```python
from build123d import *

# Parameters (mm, degrees)
F0_W      = 101.6
F0_H      = 76.2
F1_DEPTH  = 25.4
F2_R      = 6.35
F3_DEPTH  = 25.4
F4_W      = 25.4
F4_H      = 38.1
F6_W      = 30.48
F6_H      = 6.35
F8_R      = 5.08
F9_SIZE   = 5.08
F10_R     = 2.54
F11_SIZE  = 2.54
F12_SIZE  = 2.54
F13_R     = 10.3882483968
F14_DEPTH = 76.2


with BuildPart() as f1:
    # F0 (on Top) → F1 (new body)
    with BuildSketch(Plane.XY):
        Rectangle(F0_W, F0_H)
    extrude(amount=F1_DEPTH)

    # F2 (on face) → F3 (cut)
    with BuildSketch(Plane.XY.offset(25.4)):
        with Locations((-38.1, 25.4)):
            Circle(F2_R)
        with Locations((38.1, 25.4)):
            Circle(F2_R)
        with Locations((38.1, -25.4)):
            Circle(F2_R)
        with Locations((-38.1, -25.4)):
            Circle(F2_R)
    extrude(amount=-F3_DEPTH, mode=Mode.SUBTRACT)

    # F4 (on Front) → F5 (revolve)
    with BuildSketch(Plane.XZ):
        with Locations((-12.7, 44.45)):
            Rectangle(F4_W, F4_H)
    revolve(axis=Axis((0, 0, 44.45), (0, 0, 1)))

    # F6 (on Right) → F7 (revolve, cut)
    with BuildSketch(Plane.YZ):
        with Locations((-34.29, 41.275)):
            Rectangle(F6_W, F6_H)
    revolve(axis=Axis((0, 0, 63.5), (0, 0, -1)), mode=Mode.SUBTRACT)

    # F8
    f8_edges = [f1.edges().sort_by_distance(p)[0] for p in [
        (25.4, 0, 38.1),
    ]]
    fillet(f8_edges, radius=F8_R)

    # F9
    f9_edges = [f1.edges().sort_by_distance(p)[0] for p in [
        (0, -38.1, 25.4),
        (50.8, 0, 25.4),
        (0, 38.1, 25.4),
        (-50.8, 0, 25.4),
    ]]
    chamfer(f9_edges, length=F9_SIZE)

    # F10
    f10_edges = [f1.edges().sort_by_distance(p)[0] for p in [
        (25.4, 0, 25.4),
        (25.4, 0, 33.02),
        (25.4, 0, 44.45),
        (25.4, 0, 63.5),
    ]]
    fillet(f10_edges, radius=F10_R)

    # F11
    f11_edges = [f1.edges().sort_by_distance(p)[0] for p in [
        (0, -38.1, 0),
        (50.8, 0, 0),
        (0, 38.1, 0),
        (-50.8, 0, 0),
    ]]
    chamfer(f11_edges, length=F11_SIZE)

    # F12
    f12_edges = [f1.edges().sort_by_distance(p)[0] for p in [
        (-50.8, 38.1, 11.43),
        (-50.8, -38.1, 11.43),
        (50.8, 38.1, 11.43),
        (50.8, -38.1, 11.43),
    ]]
    chamfer(f12_edges, length=F12_SIZE)

    # F13 (on face) → F14 (cut)
    with BuildSketch(Plane.XY.offset(63.5)):
        Circle(F13_R)
    extrude(amount=-F14_DEPTH, mode=Mode.SUBTRACT)


solid = f1.part
```
Read the model definition and answer for the solid it produces. Units are mm, in the model's axes. A direction names the side the tool comes from. Coordinates: 2 decimals unless noted, no trailing zeros. Write each loop counter-clockwise with the first axis right and the second up, starting at its lowest first coordinate (ties: lowest second). Pieces come first, ordered by that corner, then holes. Notation, with made-up numbers: (-10.5, -14) -> (9.5, -14) arc R7 ccw to (9.5, -2) -> close; hole circle Ø2 at (74.5, -21). An arc over 180 degrees is marked (long way). Answer as a JSON object with one key per item and string values.
Q1. Consider line 1 (X direction, y = 25, z = 19); line 2 (Y direction, x = 38.1, z = 15.5); line 3 (Y direction, x = 0, z = 17.5). Determine where each line is inside the solid, lowest interval first. Write a range as [from, to].
The answers:
{"line 1": "x = [-50.8, -44.44], [-31.76, 31.76], [44.44, 50.8]", "line 2": "y = [-38.1, -31.75], [-19.05, 19.05], [31.75, 38.1]", "line 3": "y = [-38.1, -10.39], [10.39, 38.1]"}
Q2. Flat-ended cylindrical pins translate along their axes: pin 1 Ø16.5 at (x, y) = (38.1, 25.4) entering from +Z; pin 2 Ø6 at (y, z) = (-25, 49) entering from +X; pin 3 Ø5 at (x, z) = (-7, 54.5) entering from -Y; pin 4 Ø11.5 at (x, y) = (38.1, -25.4) entering from -Z. Find the tip coordinate at first contact, or state that the pin passes through.
The answers:
{"pin 1": "stops at z = 25.4", "pin 2": "stops at x = 12.69", "pin 3": "stops at y = -25", "pin 4": "passes through"}
Q3. Determine the mould class of faces 4 (the cylindrical face through (31.756, 25.679, 12.878)), 5 (the cylindrical face through (5.506, 24.796, 54.073)), 6 (the flat face through (49.51, -0.52, 1.25)) for opening direction Y: pulls with the +Y half, pulls with the -Y half, needs draft (parallel to the pull), parting line crosses it, or undercut.
The answers:
{"face 4": "undercut", "face 5": "parting line crosses it", "face 6": "needs draft"}
Q4. The part is cut by section B-B on z = 12. Give the vertices of the cut face in (x, y).
The answers:
{"outline": "(-50.8, -35.56) -> (-48.26, -38.1) -> (48.26, -38.1) -> (50.8, -35.56) -> (50.8, 35.56) -> (48.26, 38.1) -> (-48.26, 38.1) -> (-50.8, 35.56) -> close; hole circle Ø12.7 at (-38.1, -25.4); hole circle Ø12.7 at (-38.1, 25.4); hole circle Ø20.78 at (0, 0); hole circle Ø12.7 at (38.1, -25.4); hole circle Ø12.7 at (38.1, 25.4)"}
Q5. The part is cut by section C-C on x = -38.1. Give the vertices of the cut face in (y, z), then the cut area to 3 significant figures.
The answers:
{"outline": "(-38.1, 2.54) -> (-35.56, 0) -> (-31.75, 0) -> (-31.75, 25.4) -> (-33.02, 25.4) -> (-38.1, 20.32) -> close; (-19.05, 0) -> (19.05, 0) -> (19.05, 25.4) -> (-19.05, 25.4) -> close; (31.75, 0) -> (35.56, 0) -> (38.1, 2.54) -> (38.1, 20.32) -> (33.02, 25.4) -> (31.75, 25.4) -> close", "area": "1,260 mm2"}
Q6. A tool of negligible diameter and unlimited length cuts with its end or side. For faces 1 (the flat face through (-17, 9, 44.45)), 2 (the cylindrical face through (-32.234, 22.968, 12.878)), 3 (the cylindrical face through (5.506, 24.796, 30.516)), from which of +Z, -Z, +X, -X, +Y, -Y can it reach the whole face along a straight path? Write none if from no direction.
The answers:
{"face 1": "none", "face 2": "+Z, -Z", "face 3": "+Z"}
